Geometry: see drawing. Coordinates: mm, zero at the bounding-box minimum. Give positions to 0.01 mm unless a question says otherwise; leave off trailing zeros. Order: outer loops, then holes, each group sorted by start corner. A loop starts at its lowest first (then second) coordinate and runs counter-clockwise, first axis right, second up. Notation, with made-up numbers: (27.25, -8) -> (79.25, -8) arc R17 cw to (79.25, 0) -> close; hole circle Ø6 at (85, 30.25). An arc over 180 degrees is marked (long way). One line per item, written item: value. Start each with the question number.
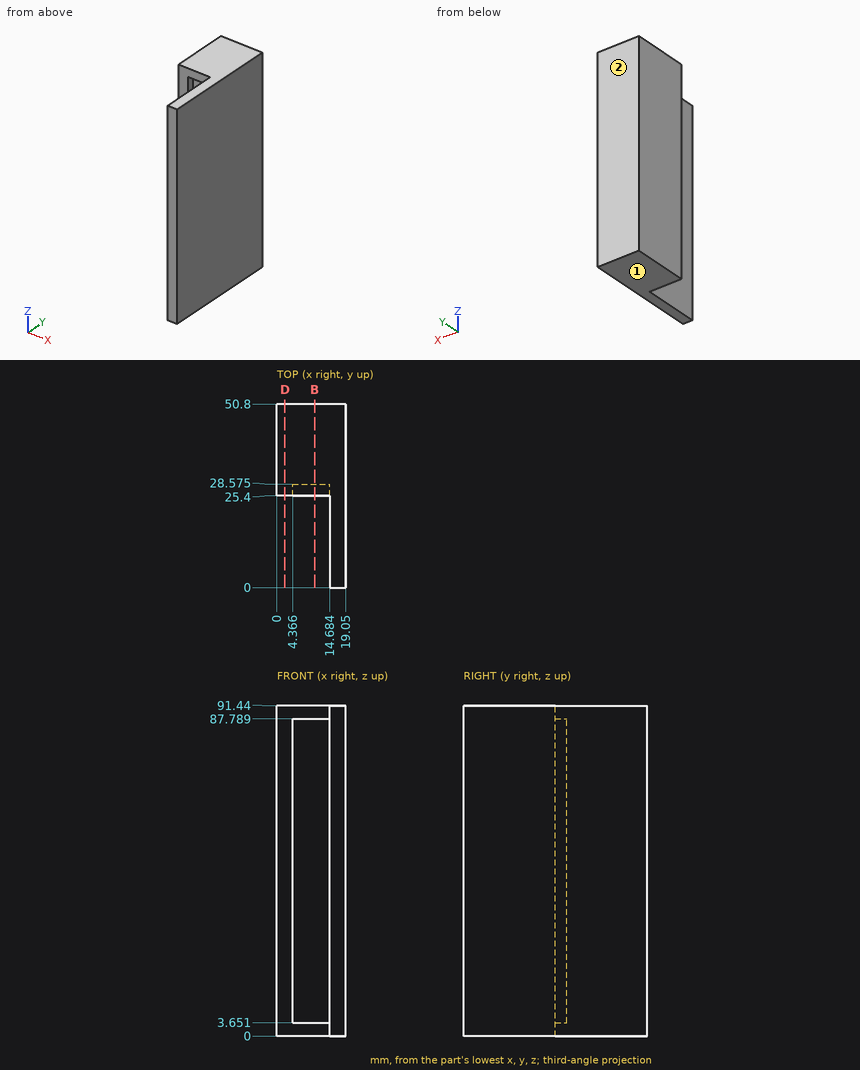
1. Material intervals for L1, parallel to Y at x = 4, z = 7; L2, parallel to Y at x = 4.5, z = 35 (1 decimal), sorted ascending. Write a range as [from, to].
2. Cut plane B-B, the plane x = 10.5. Return loops of the section in (y, z) (1 decimal), then the cut area to 3 significant figures.
3. Pin query (flat end, axial travel): P1, Ø3, axis at x = 10.5, z = 58.5, coming from the -Y side (3 decimals); P2, Ø2, axis at x = 14.5, y = 22.5, coming from the -Z side; P3, Ø8, axis at x = 4, z = 55.5, coming from the -Y side; P4, Ø10, axis at y = 15.5, z = 81, coming from the -X side. Return the tip coordinate at first contact, or that it passes through.
4. Cut plane D-D, the plane x = 2.25. Return loops of the section in (y, z), then the cut area to 3 significant figures.
5. Draft query along Y for the marked faces 1 and 2. Return one class per face: pulls with the +Y half, pulls with the -Y half, needs draft (parallel to the pull), parting line crosses it, or undercut.
Answers follow:
1. L1: y = [25.4, 50.8]
1. L2: y = [28.6, 50.8]
2. outline: (25.4, 0) -> (50.8, 0) -> (50.8, 91.4) -> (25.4, 91.4) -> (25.4, 87.8) -> (28.6, 87.8) -> (28.6, 3.7) -> (25.4, 3.7) -> close
2. area: 2,060 mm²
3. P1: stops at y = 28.575
3. P2: stops at z = 0
3. P3: stops at y = 25.4
3. P4: stops at x = 14.68
4. outline: (25.4, 0) -> (50.8, 0) -> (50.8, 91.44) -> (25.4, 91.44) -> close
4. area: 2,320 mm²
5. face 1: needs draft
5. face 2: pulls with the +Y half
